Model file for the job. Use its own axes, mm. A direction names the side the tool comes from. Round coordinates to 2 decimals unless told otherwise and drop trailing zeros. Loops run counter-clockwise (first coordinate to the right, second up) from the corner with the lowest first, then second, coordinate; pieces in that order, holes last. Notation, with made-up numbers: (53.5, 82.5) - (63.5, 82.5) arc R3 ccw to (63.5, 86.5) - close; hole circle Ø10 at (-22.75, 19.25). An arc over 180 degrees is marked (long way). Use one line per item in the form item = value.
from build123d import *

# Parameters (mm, degrees)
F0_R      = 24.305161
F1_DEPTH  = 5.08
F2_R      = 24.305161
F2_R_2    = 21.550516
F5_DEPTH  = 2.286
F4_R      = 21.550516
F4_R_2    = 17.333269
F6_DEPTH  = 1.778
F3_R      = 6.008361
F7_DEPTH  = 1.27
F8_R      = 1.480993
F9_DEPTH  = 2.54
F10_R     = 2.748389
F11_DEPTH = 25.4


with BuildPart() as f1:
    # F0 (on Front) → F1 (new body)
    with BuildSketch(Plane.XZ):
        Circle(F0_R)
    extrude(amount=F1_DEPTH)

    # F2 (on face) → F5 (join)
    with BuildSketch(Plane.XZ.offset(5.08)):
        Circle(F2_R)
        Circle(F2_R_2, mode=Mode.SUBTRACT)
    extrude(amount=F5_DEPTH)

    # F4 (on face) → F6 (join)
    with BuildSketch(Plane.XZ.offset(5.08)):
        Circle(F4_R)
        Circle(F4_R_2, mode=Mode.SUBTRACT)
    extrude(amount=F6_DEPTH)

    # F3 (on face) → F7 (join)
    with BuildSketch(Plane.XZ.offset(5.08)):
        Circle(F3_R)
    extrude(amount=F7_DEPTH)

    # F8 (on face) → F9 (join)
    with BuildSketch(Plane.XZ.offset(6.35)):
        Circle(F8_R)
    extrude(amount=F9_DEPTH)

    # F10 (on face) → F11 (cut)
    with BuildSketch(Plane.XZ.offset(5.08)):
        with Locations((0, 10.771388)):
            Circle(F10_R)
        with Locations((7.616522, 7.616522)):
            Circle(F10_R)
        with Locations((10.771388, 0)):
            Circle(F10_R)
        with Locations((7.616522, -7.616522)):
            Circle(F10_R)
        with Locations((0, -10.771388)):
            Circle(F10_R)
        with Locations((-7.616522, -7.616522)):
            Circle(F10_R)
        with Locations((-10.771388, 0)):
            Circle(F10_R)
        with Locations((-7.616522, 7.616522)):
            Circle(F10_R)
    extrude(amount=-F11_DEPTH, mode=Mode.SUBTRACT)


solid = f1.part
1. Pull direction X, two halves, no side cores. Call faces 1 (the cylindrical face through (5.591, -2.576, 9.474)), 2 (the cylindrical face through (23.183, -3.631, 7.301)), 3 (the flat face through (-15, -7.366, -16)): +X half, -X half, draft (parallel to the pull), parting line (faces both ways), or undercut.
Geometry check:
face_1 = undercut
face_2 = parting line
face_3 = draft
2. Cut at C-C, the plane y = -2.25. Give the number of separate pieces and of enclosed holes in the cut face, plus the area to 3 significant figures.
Geometry check:
separate_pieces = 1
enclosed_holes = 8
area = 1,670 mm^2
3. Cut at A-A, the plane x = 0. Give the cut face in (y, z).
Geometry check:
outline = (-8.89, -1.48) - (-6.35, -1.48) - (-6.35, -6.01) - (-5.08, -6.01) - (-5.08, -8.02) - (0, -8.02) - (0, 8.02) - (-5.08, 8.02) - (-5.08, 6.01) - (-6.35, 6.01) - (-6.35, 1.48) - (-8.89, 1.48) - close; (-7.37, -24.31) - (0, -24.31) - (0, -13.52) - (-5.08, -13.52) - (-5.08, -17.33) - (-6.86, -17.33) - (-6.86, -21.55) - (-7.37, -21.55) - close; (-7.37, 21.55) - (-6.86, 21.55) - (-6.86, 17.33) - (-5.08, 17.33) - (-5.08, 13.52) - (0, 13.52) - (0, 24.31) - (-7.37, 24.31) - close
4. Cut at D-D, the plane x = -7. Give the cut face in (y, z).
Geometry check:
outline = (-7.37, -23.28) - (0, -23.28) - (0, -10.29) - (-5.08, -10.29) - (-5.08, -15.86) - (-6.86, -15.86) - (-6.86, -20.38) - (-7.37, -20.38) - close; (-7.37, 20.38) - (-6.86, 20.38) - (-6.86, 15.86) - (-5.08, 15.86) - (-5.08, 10.29) - (0, 10.29) - (0, 23.28) - (-7.37, 23.28) - close; (-5.08, -4.94) - (0, -4.94) - (0, 4.94) - (-5.08, 4.94) - close
5. Flat gauge pins, fed straight in: pin 1 (4.5 mm diameter, centred on x = 10.77, z = 0, fed in from -Y); pin 2 (3 mm diameter, centred on y = -4, z = 5, fed in from +X); pin 3 (6.5 mm diameter, centred on x = 7.62, z = -7.62, fed in from -Y); pin 4 (5 mm diameter, centred on y = -7, z = -4, fed in from +X). Where does each tip first touch, or does it go through?
Geometry check:
pin_1 = through
pin_2 = 24.05
pin_3 = -5.08
pin_4 = 24.26
6. Tool access for faces 4 (the flat face through (0, 0, 0)), 5 (the flat face through (1, -6.858, 18)): list every direction of +Z, -Z, +X, -X, +Y, -Y with a clear straight run to the whole face (end or side of a thin tool).
Geometry check:
face_4 = +Z, -Z, +X, -X, +Y
face_5 = -Y
7. Cut at B-B, the plane z = 0. Give the cut face in (x, y).
Geometry check:
outline = (-24.31, -7.37) - (-21.55, -7.37) - (-21.55, -6.86) - (-17.33, -6.86) - (-17.33, -5.08) - (-13.52, -5.08) - (-13.52, 0) - (-24.31, 0) - close; (-8.02, -5.08) - (-6.01, -5.08) - (-6.01, -6.35) - (-1.48, -6.35) - (-1.48, -8.89) - (1.48, -8.89) - (1.48, -6.35) - (6.01, -6.35) - (6.01, -5.08) - (8.02, -5.08) - (8.02, 0) - (-8.02, 0) - close; (13.52, -5.08) - (17.33, -5.08) - (17.33, -6.86) - (21.55, -6.86) - (21.55, -7.37) - (24.31, -7.37) - (24.31, 0) - (13.52, 0) - close
8. Wall check: probe 1 along Z at (x, y) = (0, -6.2); probe 2 along Z at (x, y) = (0, -2.15); probe 3 along Z at (x, y) = (8.5, -4.75). Give the ranges that are in metal, low to high.
Geometry check:
probe_1 = -24.31 to -17.33, -6.01 to 6.01, 17.33 to 24.31
probe_2 = -24.31 to -13.52, -8.02 to 8.02, 13.52 to 24.31
probe_3 = -22.77 to -10.22, -5.01 to -1.55, 1.55 to 5.01, 10.22 to 22.77
